from build123d import *

# Parameters (mm, degrees)
SKETCH1_R               = 5
BOSS_EXTRUDE1_DEPTH     = 24.9
SKETCH2_R               = 2.925
BOSS_EXTRUDE2_DEPTH     = 8.1
FILLET1_R               = 1.5
CUT_EXTRUDE1_DEPTH      = 34.749074061
CUT_EXTRUDE1_DEPTH_BACK = 34.749074061
SKETCH3_R               = 1.175
SKETCH4_R               = 1.25
CUT_EXTRUDE2_DEPTH      = 10


with BuildPart() as part:
    # Sketch1 → Boss-Extrude1 (new body)
    with BuildSketch(Plane(origin=(0, 0, 0), x_dir=(1, 0, 0), z_dir=(0, 1, 0))):
        with Locations(Location((0, 0, 0), (0, 0, 270))):
            Circle(SKETCH1_R)
    extrude(amount=BOSS_EXTRUDE1_DEPTH)

    # Sketch2 → Boss-Extrude2 (add)
    with BuildSketch(Plane(origin=(0, 24.9, 0), x_dir=(1, 0, 0), z_dir=(0, 1, 0))):
        with Locations(Location((0, 0, 0), (0, 0, 90))):
            Circle(SKETCH2_R)
    extrude(amount=BOSS_EXTRUDE2_DEPTH)

    # Fillet1
    fillet1_edges = [part.edges().sort_by_distance(p)[0] for p in [
        (0, 33, 2.925),
    ]]
    fillet(fillet1_edges, radius=FILLET1_R)

    # Sketch3 → Cut-Extrude1 (cut, two sides: drawn at the far end of the back side and taken through both)
    with BuildSketch(Plane(origin=(0, 0, 0), x_dir=(0, 0, -1), z_dir=(1, 0, 0)).offset(-CUT_EXTRUDE1_DEPTH_BACK)):
        with Locations((0, 28.66)):
            Circle(SKETCH3_R)
    extrude(amount=CUT_EXTRUDE1_DEPTH + CUT_EXTRUDE1_DEPTH_BACK, mode=Mode.SUBTRACT)

    # Sketch4 → Cut-Extrude2 (cut)
    with BuildSketch(Plane.XZ):
        with Locations(Location((0, 0, 0), (0, 0, 270))):
            Circle(SKETCH4_R)
    extrude(amount=-CUT_EXTRUDE2_DEPTH, mode=Mode.SUBTRACT)


solid = part.part
Here's how the part is built. I have some questions about the finished solid (model axes, mm). A direction names the side the tool comes from. Give positions to 0.01 mm unless a question says otherwise; leave off trailing zeros. Loops run counter-clockwise (first coordinate to the right, second up) from the corner with the lowest first, then second, coordinate; pieces in that order, holes last. Notation, with made-up numbers: (48.25, 9.5) -> (66.25, 9.5) arc R26 cw to (66.25, 46.5) -> close; hole circle Ø1 at (-27, -27.5). An arc over 180 degrees is marked (long way). Answer as a JSON object with one key per item and string values. Group by question number.
Item 1: Will these pins go through, and if not, where does the flat tip stop? pin 1 (1.5 mm diameter, centred on x = 0, z = 3, fed in from +Y); pin 2 (1.2 mm diameter, centred on x = 0, z = 0, fed in from -Y); pin 3 (5 mm diameter, centred on y = 28, z = -3, fed in from +X).
Item 2: Imagine slicing it at D-D on y = 28.66. Write out the boundary of the cut face in (x, z) (3 decimals), then the cut area to 3 significant figures.
Item 3: Thinking about a two-plate mould opening in Z: for faces 1 (the cylindrical face through (-4.88, 12.28, -1.08)), 2 (the flat face through (-2.2, 24.9, 2.2)), 3 (the flat face through (0, 10, 0)), which applies, pulls with the +Z half, pulls with the -Z half, needs draft (parallel to the pull), parting line crosses it, or undercut?
Item 4: Imagine slicing it at B-B on x = -4. Write out the boundary of the cut face in (y, z).
Item 5: Imagine slicing it at A-A on y = 6. Write out the boundary of the cut face in (x, z), then the cut area to 3 significant figures.
Item 6: I need wall thicknesses on L1, parallel to Y at x = 0.25, z = 0 (3 decimals); L2, parallel to X at y = 5.5, z = 0; L3, parallel to Y at x = -1, z = 3. Which ranges of each line are inside material? Lowest first, please.
Item 7: Imagine slicing it at C-C on y = 16. Write out the boundary of the cut face in (x, z), then the cut area to 3 significant figures.
Item 8: On a 3-axis mill with a long thin cutter (end or side, diameter ignored), from which of +Z, -Z, +X, -X, +Y, -Y can I reach the whole of each face in a straight line? I mean faces 4 (the cylindrical face through (-1.22, 4.93, 0.27)), 5 (the flat face through (-1, 0, 1)), 6 (the cylindrical face through (1.12, 28.15, -2.7)). Say none if no direction works.
Answer list:
{
 "1": {"pin 1": "stops at y = 32.75", "pin 2": "stops at y = 10", "pin 3": "stops at x = 2.88"},
 "2": {"outline": "(-2.679, -1.175) arc R2.925 ccw to (2.679, -1.175) -> close; (-2.679, 1.175) -> (2.679, 1.175) arc R2.925 ccw to start", "area": "13.5 mm2"},
 "3": {"face 1": "parting line crosses it", "face 2": "needs draft", "face 3": "undercut"},
 "4": {"outline": "(0, -3) -> (24.9, -3) -> (24.9, 3) -> (0, 3) -> close"},
 "5": {"outline": "circle Ø10 at (0, 0); hole circle Ø2.5 at (0, 0)", "area": "73.6 mm2"},
 "6": {"L1": "y = 10 to 27.485, 29.835 to 33", "L2": "x = -5 to -1.25, 1.25 to 5", "L3": "y = 0 to 24.9"},
 "7": {"outline": "circle Ø10 at (0, 0)", "area": "78.5 mm2"},
 "8": {"face 4": "-Y", "face 5": "+Z, -Z, +X, -X, -Y", "face 6": "+Y"}
}
